Autodesk Inventor part; units mm, degrees
ref_plane "NUT_XY" through (0, 0, 0) normal (0, 0, 1) x (1, 0, 0)
ref_plane "NUT_YZ" through (0, 0, 0) normal (1, 0, 0) x (0, 1, 0)
ref_plane "NUT_ZX" through (0, 0, 0) normal (0, 1, 0) x (0, 0, 1)
sketch "Sketch_8" plane through (0, 0, 0) normal (1, 0, 0) x (0, 1, 0)
  line L0 (0, -5.588) -> (0, 0)
  line L1 (0, 0) -> (7.112, 0)
  line L2 (7.112, 0) -> (8.5344, -0.3811)
  line L3 (8.5344, -0.3811) -> (8.5344, -5.2069)
  line L4 (8.5344, -5.2069) -> (7.112, -5.588)
  line L5 (7.112, -5.588) -> (0, -5.588)
  line L6 (0, -5.588) -> (0, 0)
sketch "Sketch_10" plane through (0, 0, 0) normal (0, 0, 1) x (1, 0, 0)
  line L0 (-14.224, 14.224) -> (-14.224, -14.224)
  line L1 (-14.224, -14.224) -> (14.224, -14.224)
  line L2 (14.224, -14.224) -> (14.224, 14.224)
  line L3 (14.224, 14.224) -> (-14.224, 14.224)
  line L4 (-7.112, 4.1061) -> (-7.112, -4.1061)
  line L5 (-7.112, -4.1061) -> (0, -8.2122)
  line L6 (0, -8.2122) -> (7.112, -4.1061)
  line L7 (7.112, -4.1061) -> (7.112, 4.1061)
  line L8 (7.112, 4.1061) -> (0, 8.2122)
  line L9 (0, 8.2122) -> (-7.112, 4.1061)
revolve "Revolution1" add sketch "Sketch_8" angle 360 about axis through (0, 0, -5.588) along (0, 0, -1)
extrude "Extrusion1" cut sketch "Sketch_10" against normal blind 5.588
sketch "Sketch_11" plane through (0, 0, 0) normal (1, 0, 0) x (0, 1, 0)
  line L0 (0, -5.588) -> (0, 0)
  line L1 (0, 0) -> (4.7625, 0)
  line L2 (4.7625, 0) -> (4.1897, -0.5728)
  line L3 (4.1897, -0.5728) -> (4.1897, -5.0152)
  line L4 (4.1897, -5.0152) -> (4.7625, -5.588)
  line L5 (4.7625, -5.588) -> (0, -5.588)
  line L6 (0, -5.588) -> (0, 0)
revolve "Revolution2" cut sketch "Sketch_11" angle 360 about axis through (0, 0, -5.588) along (0, 0, -1)
thread "Thread1"
ref_plane "NUT_XY" through (0, 0, 0) normal (0, 0, 1) x (1, 0, 0)
ref_plane "NUT_YZ" through (0, 0, 0) normal (1, 0, 0) x (0, 1, 0)
ref_plane "NUT_ZX" through (0, 0, 0) normal (0, 1, 0) x (0, 0, 1)
ref_plane "a1_XY" through (-7.112, 7.112, 0) normal (0, 0, 1) x (1, 0, 0)
ref_plane "a1_YZ" through (-7.112, 7.112, 0) normal (1, 0, 0) x (0, 1, 0)
ref_plane "a1_ZX" through (-7.112, 7.112, 0) normal (0, 1, 0) x (0, 0, 1)
ref_plane "a2_XY" through (7.112, 7.112, 0) normal (0, 0, 1) x (1, 0, 0)
ref_plane "a2_YZ" through (7.112, 7.112, 0) normal (1, 0, 0) x (0, 1, 0)
ref_plane "a2_ZX" through (7.112, 7.112, 0) normal (0, 1, 0) x (0, 0, 1)
ref_plane "b1_XY" through (0, 7.112, 0) normal (1, 0, 0) x (0, 0, -1)
ref_plane "b1_YZ" through (0, 7.112, 0) normal (0, 0, -1) x (0, 1, 0)
ref_plane "b1_ZX" through (0, 7.112, 0) normal (0, 1, 0) x (1, 0, 0)
ref_plane "b2_XY" through (0, 7.112, -5.588) normal (1, 0, 0) x (0, 0, -1)
ref_plane "b2_YZ" through (0, 7.112, -5.588) normal (0, 0, -1) x (0, 1, 0)
ref_plane "b2_ZX" through (0, 7.112, -5.588) normal (0, 1, 0) x (1, 0, 0)
ref_plane "e_XY" through (0, 0, -5.588) normal (1, 0, 0) x (0, 0, -1)
ref_plane "e_YZ" through (0, 0, -5.588) normal (0, 0, -1) x (0, 1, 0)
ref_plane "e_ZX" through (0, 0, -5.588) normal (0, 1, 0) x (1, 0, 0)
ref_plane "th1_XY" through (0, 4.7625, -5.588) normal (1, 0, 0) x (0, 0, -1)
ref_plane "th1_YZ" through (0, 4.7625, -5.588) normal (0, 0, -1) x (0, 1, 0)
ref_plane "th1_ZX" through (0, 4.7625, -5.588) normal (0, 1, 0) x (1, 0, 0)
ref_plane "th2_XY" through (0, -4.7625, -5.588) normal (1, 0, 0) x (0, 0, -1)
ref_plane "th2_YZ" through (0, -4.7625, -5.588) normal (0, 0, -1) x (0, 1, 0)
ref_plane "th2_ZX" through (0, -4.7625, -5.588) normal (0, 1, 0) x (1, 0, 0)
ref_plane "ol1_XY" through (0, 0, -7.112) normal (0, 1, 0) x (1, 0, 0)
ref_plane "ol1_YZ" through (0, 0, -7.112) normal (1, 0, 0) x (0, 0, -1)
ref_plane "ol1_ZX" through (0, 0, -7.112) normal (0, 0, -1) x (0, 1, 0)
ref_plane "ol2_XY" through (5.588, 0, -7.112) normal (0, 1, 0) x (1, 0, 0)
ref_plane "ol2_YZ" through (5.588, 0, -7.112) normal (1, 0, 0) x (0, 0, -1)
ref_plane "ol2_ZX" through (5.588, 0, -7.112) normal (0, 0, -1) x (0, 1, 0)
properties part number "D-801"
Verification items for the finished model (mm, model axes). Round coordinates to 2 decimals unless told otherwise and drop trailing zeros. Loops run counter-clockwise (first coordinate to the right, second up) from the corner with the lowest first, then second, coordinate; pieces in that order, holes last. Notation, with made-up numbers: (36.5, 51.5) - (49.5, 51.5) arc R24 ccw to (49.5, 72.5) - close; hole circle Ø1 at (35.25, 72.25). An arc over 180 degrees is marked (long way). Answer in a Markdown table with one row per item. Add a question column.
Q1. Gauge pin test, flat ends, axial feed: pin 1 (5 mm diameter, centred on x = 0, y = 1, fed in from -Z); pin 2 (1 mm diameter, centred on x = 4, z = -3, fed in from +Y); pin 3 (2 mm diameter, centred on x = 5.5, z = -3, fed in from +Y). Record the tip position at first contact, or that the pin passes through.
Q2. Material ranges on line 1 (X direction, y = 0, z = -3.15); line 2 (Y direction, x = -0.25, z = -3.35); line 3 (X direction, y = -2.5, z = -1.7), recorded low to high.
Q3. Release check for a two-part mould opening along Y. For faces 1 (the face through (-0.02, 7.34, -0.06)), 2 (the face through (-4.09, -0.91, -2.83)), 3 (the face through (-7.112, 0, -3)), 4 (the face through (3.506, -6.188, -2.755)) record: pulls with the +Y half, pulls with the -Y half, needs draft (parallel to the pull), parting line crosses it, or undercut.
Q4. Section check A-A on z = -4.55. Enter the section's corners in (x, y), plus the area to 3 significant figures.
Found:
| question | item | result |
|---|---|---|
| 1 | pin 1 | passes through |
| 1 | pin 2 | stops at y = 6.19 |
| 1 | pin 3 | stops at y = 5.61 |
| 2 | line 1 | x = -7.11 to -4.19, 4.19 to 7.11 |
| 2 | line 2 | y = -8.07 to -4.18, 4.18 to 8.07 |
| 2 | line 3 | x = -7.11 to -3.36, 3.36 to 7.11 |
| 3 | face 1 | pulls with the +Y half |
| 3 | face 2 | undercut |
| 3 | face 3 | needs draft |
| 3 | face 4 | pulls with the -Y half |
| 4 | outline | (-7.11, -4.11) - (0, -8.21) - (7.11, -4.11) - (7.11, 4.11) - (0, 8.21) - (-7.11, 4.11) - close; hole circle Ø8.38 at (0, 0) |
| 4 | area | 120 mm² |
